from build123d import *


with BuildPart() as part:
    # Sketch2 → Revolve1 (revolve)
    with BuildSketch(Plane(origin=(0, 0, 0), x_dir=(0, 0, -1), z_dir=(1, 0, 0))):
        with BuildLine():
            Line((30, 0), (-30, 0))
            Line((-30, 0), (-12.5, 17.5))
            Line((-12.5, 17.5), (-12.5, 62.5))
            Line((-12.5, 62.5), (-30, 80))
            ThreePointArc((-30, 80), (0, 110), (30, 80))
            Line((30, 80), (12.5, 62.5))
            Line((12.5, 62.5), (12.5, 17.5))
            Line((12.5, 17.5), (30, 0))
        make_face()
    revolve(axis=Axis((0, 0, -30), (0, 0, 1)))


solid = part.part
Model file for the job. Use its own axes, mm. A direction names the side the tool comes from. Coordinates: 2 decimals unless noted, no trailing zeros. Order: outer loops, then holes, each group sorted by start corner. A loop starts at its lowest first (then second) coordinate and runs counter-clockwise, first axis right, second up. Notation, with made-up numbers: (-27.75, -7.5) -> (-22.75, -7.5) arc R23 cw to (-22.75, 18.5) -> close; hole circle Ø9 at (75.5, 89.25). An arc over 180 degrees is marked (long way). Return JSON: item names as keys, results as strings. Group by question number.
Item 1: Wall check: line 1 along Z through (x, y) = (39, 31); line 2 along Y through (x, z) = (5.5, 16); line 3 along Y through (x, z) = (31.5, 17.5). Give the ranges that are in metal, low to high. Write a range as [from, to].
Item 2: Flat gauge pins, fed straight in: P1, Ø10, axis at x = 58, y = -28, coming from the -Z side; P2, Ø12, axis at x = 73, z = -12, coming from the -Y side; P3, Ø10, axis at x = 44.5, z = 9, coming from the +Y side. Where does each tip first touch, or does it go through?
Item 3: Saw through at A-A on z = 9. Write the cut outline in (x, y).
Item 4: Tool access for faces 1 (the flat face through (13, -13, 12.5)), 2 (the flat face through (13, 13, -12.5)): list every direction of +Z, -Z, +X, -X, +Y, -Y with a clear straight run to the whole face (end or side of a thin tool).
Values found:
{
 "1": {"line 1": "z = [-12.5, 12.5]", "line 2": "y = [-105.23, -65.77], [-12.87, 12.87], [65.77, 105.23]", "line 3": "y = [-99.5, -59.7], [59.7, 99.5]"},
 "2": {"P1": "stops at z = -19.4", "P2": "stops at y = -84.86", "P3": "stops at y = 101.64"},
 "3": {"outline": "circle Ø217.24 at (0, 0)"},
 "4": {"face 1": "+Z", "face 2": "-Z"}
}
